Could you check a few things on this model? Use its own coordinates, in mm. Face numbers are marked on the shaded views. A direction names the side the tool comes from. Give positions to 0.01 mm unless a question says otherwise; leave off trailing zeros. Loops run counter-clockwise (first coordinate to the right, second up) from the corner with the lowest first, then second, coordinate; pieces in that order, holes last. Notation, with made-up numbers: (57, 45.25) -> (97, 45.25) arc R29 cw to (97, 76.25) -> close; hole circle Ø7 at (-27, 71.5). An arc over 180 degrees is marked (long way). Put each result on its own line as item: value.
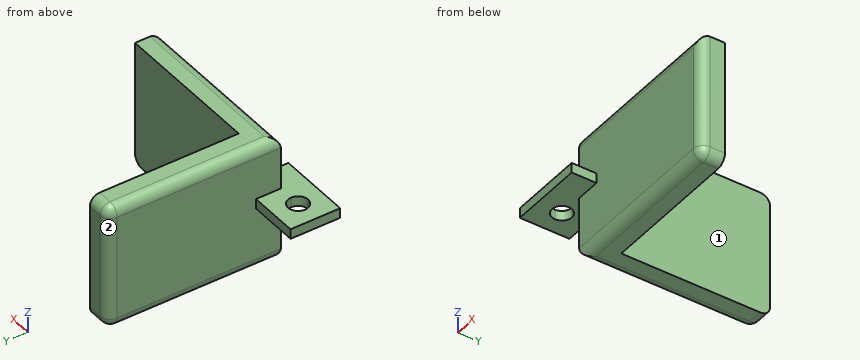
```python
from build123d import *

# Parameters (mm, degrees)
F1_DEPTH = 25
F2_W     = 5
F2_H     = 2
F3_DEPTH = 5
F5_DEPTH = 10
F7_DEPTH = 25
F8_R     = 2


with BuildPart() as f1:
    # F0 (on Top) → F1 (new body)
    with BuildSketch(Plane.XY):
        Polygon((0, -5), (0, 0), (-30, 0), (-30, 30), (-35, 30), (-35, -5), align=None)
    extrude(amount=F1_DEPTH)

    # F2 (on face) → F3 (join)
    with BuildSketch(Plane.XZ.offset(5)):
        with Locations((-32.5, 13.5)):
            Rectangle(F2_W, F2_H)
    extrude(amount=F3_DEPTH)

    # F4 (on face) → F5 (join)
    with BuildSketch(Plane(origin=(-35, 0, 0), x_dir=(0, -1, 0), z_dir=(-1, 0, 0))):
        Polygon((10, 14.5), (5, 14.5), (0, 14.5), (0, 12.5), (5, 12.5), (10, 12.5), align=None)
    extrude(amount=F5_DEPTH)

    # F6 (on face) → F7 (cut)
    with BuildSketch(Plane.XY.offset(14.5)):
        with BuildLine():
            Line((-40, -7), (-40, -5))
            Line((-40, -5), (-41.4142135624, -6.4142135624))
            ThreePointArc((-41.4142135624, -6.4142135624), (-40.7653668647, -6.847759065), (-40, -7))
        make_face()
        with BuildLine():
            ThreePointArc((-40, -7), (-38.5857864376, -6.4142135624), (-38, -5))
            Line((-38, -5), (-40, -5))
            Line((-40, -5), (-40, -7))
        make_face()
        with BuildLine():
            Line((-40, -5), (-38, -5))
            ThreePointArc((-38, -5), (-38.5857864376, -3.5857864376), (-40, -3))
            Line((-40, -3), (-40, -5))
        make_face()
        with BuildLine():
            Line((-42, -5), (-40, -5))
            Line((-40, -5), (-40, -3))
            ThreePointArc((-40, -3), (-41.4142135624, -3.5857864376), (-42, -5))
        make_face()
        with BuildLine():
            Line((-41.4142135624, -6.4142135624), (-40, -5))
            Line((-40, -5), (-42, -5))
            ThreePointArc((-42, -5), (-41.847759065, -5.7653668647), (-41.4142135624, -6.4142135624))
        make_face()
    extrude(amount=-F7_DEPTH, mode=Mode.SUBTRACT)

    # F8
    f8_edges = [f1.edges().sort_by_distance(p)[0] for p in [
        (-35, 12.5, 0),
        (-17.5, -5, 0),
        (0, -2.5, 0),
        (-32.5, 30, 0),
        (-35, 30, 12.5),
        (-35, 12.5, 25),
        (-32.5, 30, 25),
        (-17.5, -5, 25),
        (0, -5, 12.5),
    ]]
    fillet(f8_edges, radius=F8_R)


solid = f1.part
```
1. For the marked faces 1 and 2, which set-ups out of +Z, -Z, +X, -X, +Y, -Y let a thin tool reach every point of the face, with its end or its side?
Recorded:
face 1: +Z, -Z, +X, +Y
face 2: +Z, -Z, -X, +Y
2. I'm going to push flat-ended pins straight in: pin 1 (1.6 mm diameter, centred on x = -41.5, z = 13.5, fed in from +Y); pin 2 (6 mm diameter, centred on x = -36.5, z = 13, fed in from +Y); pin 3 (5 mm diameter, centred on x = -36, y = -3.5, fed in from -Z). Where does each tip first touch, or does it pass through?
Recorded:
pin 1: stops at y = 0
pin 2: stops at y = 29.94
pin 3: stops at z = 0.06
3. If we section it at D-D (x = -4): List the corners of the cut face in (y, z) for me.
Recorded:
outline: (-5, 2) arc R2 ccw to (-3, 0) -> (0, 0) -> (0, 25) -> (-3, 25) arc R2 ccw to (-5, 23) -> close
4. If we section it at A-A (z = 13.75): List the corners of the cut face in (x, y) for me, then the cut area to 3 significant figures.
Recorded:
outline: (-45, -10) -> (-30, -10) -> (-30, -5) -> (-2, -5) arc R2 ccw to (0, -3) -> (0, 0) -> (-30, 0) -> (-30, 30) -> (-33, 30) arc R2 ccw to (-35, 28) -> (-35, 0) -> (-45, 0) -> close; hole circle Ø4 at (-40, -5)
area: 436 mm^2
5. I need wall thicknesses on line 1 (X direction, y = 26, z = 19); line 2 (Y direction, x = -13, z = 17); line 3 (X direction, y = -4, z = 13.75). Which ranges of each line are inside material? Lowest first, please.
Recorded:
line 1: x = -35 to -30
line 2: y = -5 to 0
line 3: x = -45 to -41.73, -38.27 to -0.27
6. If we section it at C-C (y = 25.5): List the corners of the cut face in (x, z) for me.
Recorded:
outline: (-35, 2) arc R2 ccw to (-33, 0) -> (-30, 0) -> (-30, 25) -> (-33, 25) arc R2 ccw to (-35, 23) -> close
7. If we section it at B-B (z = 21.75): List the corners of the cut face in (x, y) for me, then the cut area to 3 significant figures.
Recorded:
outline: (-35, -5) -> (-2, -5) arc R2 ccw to (0, -3) -> (0, 0) -> (-30, 0) -> (-30, 30) -> (-33, 30) arc R2 ccw to (-35, 28) -> close
area: 323 mm^2
